Input: part model. Units: mm. Frame: model coordinates. Face numbers are marked on the shaded views. Round coordinates to 2 decimals unless told otherwise and drop trailing zeros. Order: outer loops, then holes, each group sorted by start corner. A loop starts at its lowest first (then second) coordinate and runs counter-clockwise, first axis right, second up.
Item 1: Cut plane A-A on x = 0. Output: boundary loops of the cut face in (y, z).
Item 2: Cut plane D-D on z = 8.5. Output: boundary loops of the cut face in (x, y), then the cut area to 3 significant figures.
Item 3: Mould query, pull axis X, two halves, no side actions, for the marked faces 1, 2 and 3. Classes: released by +X, released by -X, zero draft, split by the parting line, or undercut.
Item 4: Cut plane B-B on y = 0. Output: boundary loops of the cut face in (x, z), then the cut area to 3 significant figures.
Item 5: Cut plane C-C on x = 11. Output: boundary loops of the cut face in (y, z).
Item 6: First-contact query: pin 1 (4 mm diameter, centred on x = -23.5, z = 1.5, fed in from -Y); pin 2 (7 mm diameter, centred on x = 22, y = 0, fed in from -Z); pin 3 (3.5 mm diameter, centred on x = -11, y = -19.05, fed in from +Z); pin 4 (8 mm diameter, centred on x = -2, y = -1, fed in from -Z). Flat tips, straight axial feed; report the tip coordinate or a pass-through.
Item 7: Line query: L1, parallel to X at y = -2, z = 5.25; L2, parallel to X at y = -20, z = 5; L3, parallel to Y at x = -11, z = 3. Output: solid intervals per line, ascending.
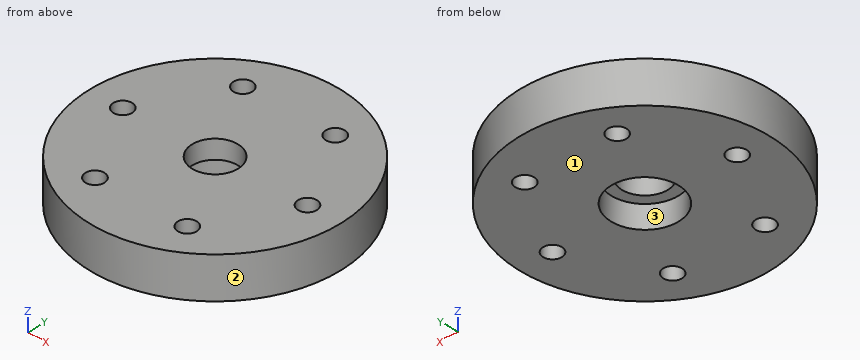
```python
from build123d import *

# Parameters (mm, degrees)
ESQUISSE1_R        = 30.1
ESQUISSE1_R_2      = 2.25
ESQUISSE1_R_3      = 8.1
BOSS_EXTRU_1_DEPTH = 10
BOSS_EXTRU_2_START = -4.5
ESQUISSE2_R        = 8.1
ESQUISSE2_R_2      = 5.5
BOSS_EXTRU_2_DEPTH = 4.5


with BuildPart() as part:
    # Esquisse1 → Boss.-Extru.1 (new body)
    with BuildSketch(Plane.XY):
        Circle(ESQUISSE1_R)
        with Locations((22, 0)):
            Circle(ESQUISSE1_R_2, mode=Mode.SUBTRACT)
        with Locations((11, -19.052558883)):
            Circle(ESQUISSE1_R_2, mode=Mode.SUBTRACT)
        with Locations((-11, -19.052558883)):
            Circle(ESQUISSE1_R_2, mode=Mode.SUBTRACT)
        with Locations((-22, 0)):
            Circle(ESQUISSE1_R_2, mode=Mode.SUBTRACT)
        with Locations((-11, 19.052558883)):
            Circle(ESQUISSE1_R_2, mode=Mode.SUBTRACT)
        with Locations((11, 19.052558883)):
            Circle(ESQUISSE1_R_2, mode=Mode.SUBTRACT)
        Circle(ESQUISSE1_R_3, mode=Mode.SUBTRACT)
    extrude(amount=BOSS_EXTRU_1_DEPTH)

    # Esquisse2 → Boss.-Extru.2 (add)
    with BuildSketch(Plane.XY.offset(10).offset(BOSS_EXTRU_2_START)):
        Circle(ESQUISSE2_R)
        Circle(ESQUISSE2_R_2, mode=Mode.SUBTRACT)
    extrude(amount=BOSS_EXTRU_2_DEPTH)


solid = part.part
```
From the geometry:
1. outline: (-30.1, 0) - (-8.1, 0) - (-8.1, 5.5) - (-5.5, 5.5) - (-5.5, 10) - (-30.1, 10) - close; (5.5, 5.5) - (8.1, 5.5) - (8.1, 0) - (30.1, 0) - (30.1, 10) - (5.5, 10) - close
2. outline: circle Ø60.2 at (0, 0); hole circle Ø4.5 at (-22, 0); hole circle Ø4.5 at (-11, -19.05); hole circle Ø4.5 at (-11, 19.05); hole circle Ø11 at (0, 0); hole circle Ø4.5 at (11, -19.05); hole circle Ø4.5 at (11, 19.05); hole circle Ø4.5 at (22, 0)
2. area: 2,660 mm2
3. face 1: zero draft
3. face 2: split by the parting line
3. face 3: undercut
4. outline: (-30.1, 0) - (-24.25, 0) - (-24.25, 10) - (-30.1, 10) - close; (-19.75, 0) - (-8.1, 0) - (-8.1, 5.5) - (-5.5, 5.5) - (-5.5, 10) - (-19.75, 10) - close; (5.5, 5.5) - (8.1, 5.5) - (8.1, 0) - (19.75, 0) - (19.75, 10) - (5.5, 10) - close; (24.25, 0) - (30.1, 0) - (30.1, 10) - (24.25, 10) - close
4. area: 373 mm2
5. outline: (-28.02, 0) - (-21.3, 0) - (-21.3, 10) - (-28.02, 10) - close; (-16.8, 0) - (16.8, 0) - (16.8, 10) - (-16.8, 10) - close; (21.3, 0) - (28.02, 0) - (28.02, 10) - (21.3, 10) - close
6. pin 1: stops at y = -21.07
6. pin 2: stops at z = 0
6. pin 3: passes through
6. pin 4: stops at z = 5.5
7. L1: x = -30.03 to -23.03, -20.97 to -7.85, 7.85 to 20.97, 23.03 to 30.03
7. L2: x = -22.49 to -13.04, -8.96 to 8.96, 13.04 to 22.49
7. L3: y = -28.02 to -21.3, -16.8 to 16.8, 21.3 to 28.02
